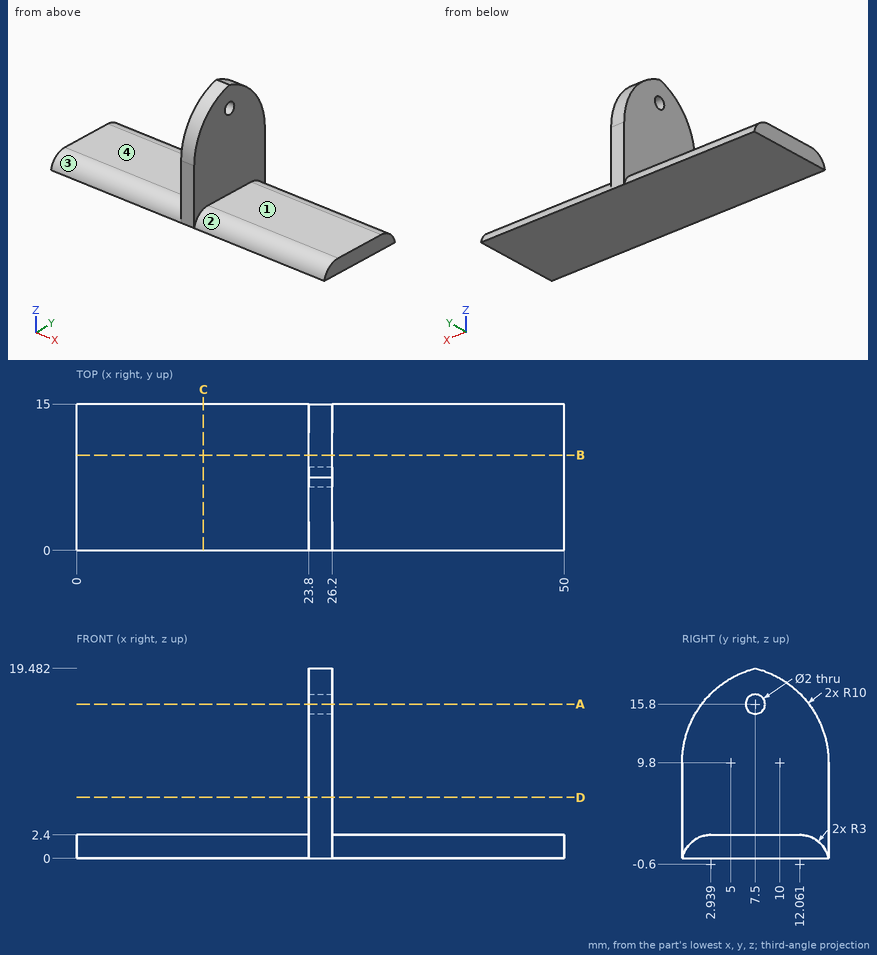
Geometry: see drawing. Coordinates: mm, zero at the bounding-box minimum. A direction names the side the tool comes from. Coordinates: 2 decimals unless noted, no trailing zeros. Loops run counter-clockwise (first coordinate to the right, second up) from the corner with the lowest first, then second, coordinate; pieces in that order, holes last. Notation, with made-up numbers: (-25.5, 4.5) -> (18.5, 4.5) arc R4 ccw to (18.5, 8.5) -> close; hole circle Ø9 at (45.5, 51.5). An arc over 180 degrees is marked (long way). Use a Markdown table: item, result.
1) Cut plane D-D (z = 6.25). Return the cut outline in (x, y), then the cut area to 3 significant figures.
Results found:
| item | result |
|---|---|
| outline | (23.8, 0) -> (26.2, 0) -> (26.2, 15) -> (23.8, 15) -> close |
| area | 36.0 mm2 |
2) Contact query for flat-ended pins moving along their axis: pin 1 (8 mm diameter, centred on x = 9, y = 4.5, fed in from +Z); pin 2 (2.5 mm diameter, centred on y = 7.5, z = 15.8, fed in from -X); pin 3 (8 mm diameter, centred on x = 22, y = 5, fed in from +Z). Output: stop coordinate, or through.
Results found:
| item | result |
|---|---|
| pin 1 | stops at z = 2.4 |
| pin 2 | stops at x = 23.8 |
| pin 3 | stops at z = 19.48 |
3) Material intervals for line 1 along Z through (x, y) = (24.8, 7.5); line 2 along X through (y, z) = (9.75, 16.75); line 3 along Z through (x, y) = (6.5, 11.5), sorted ascending. Write a range as from..to.
Results found:
| item | result |
|---|---|
| line 1 | z = 0..14.8, 16.8..19.48 |
| line 2 | x = 23.8..26.2 |
| line 3 | z = 0..2.4 |
4) Cut plane A-A (z = 15.8). Return the cut outline in (x, y).
Results found:
| item | result |
|---|---|
| outline | (23.8, 2) -> (26.2, 2) -> (26.2, 6.5) -> (23.8, 6.5) -> close; (23.8, 8.5) -> (26.2, 8.5) -> (26.2, 13) -> (23.8, 13) -> close |
5) Cut plane B-B (y = 9.75). Return the cut outline in (x, z), then the cut area to 3 significant figures.
Results found:
| item | result |
|---|---|
| outline | (0, 0) -> (50, 0) -> (50, 2.4) -> (26.2, 2.4) -> (26.2, 18.6) -> (23.8, 18.6) -> (23.8, 2.4) -> (0, 2.4) -> close |
| area | 159 mm2 |
6) Cut plane C-C (x = 13). Return the cut outline in (y, z).
Results found:
| item | result |
|---|---|
| outline | (0, 0) -> (15, 0) arc R3 ccw to (12.06, 2.4) -> (2.94, 2.4) arc R3 ccw to start |
7) Access query for the marked faces 1, 2, 3 and 4. Directions: +Z, -Z, +X, -X, +Y, -Y. A direction counts if a zero-diameter tool reaches every point of the face in a straight line with its end or side. Return the directions, or none.
Results found:
| item | result |
|---|---|
| face 1 | +Z, +X, +Y, -Y |
| face 2 | +Z, +X, -Y |
| face 3 | +Z, -X, -Y |
| face 4 | +Z, -X, +Y, -Y |
